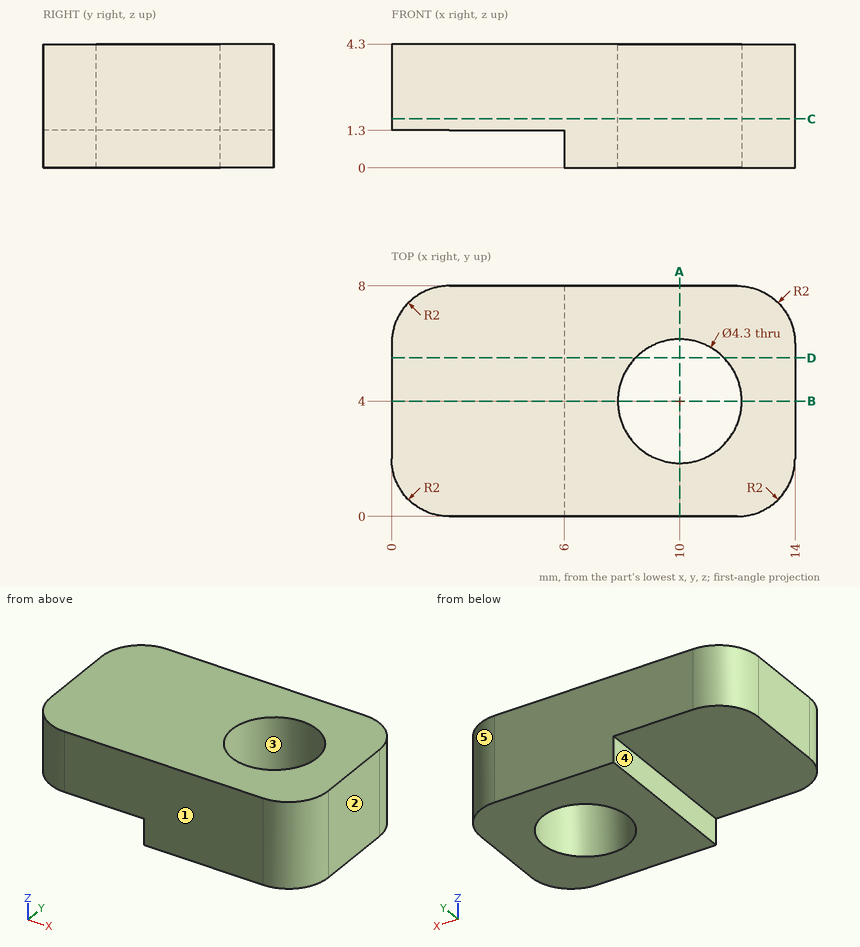
Design review of the part shown in the three views and the two pictorial views. Dimensions are in mm from the part's minimum x, y and z. A direction names the side the tool comes from. Give positions to 0.01 mm unless a question says otherwise; leave off trailing zeros. Loops run counter-clockwise (first coordinate to the right, second up) from the corner with the lowest first, then second, coordinate; pieces in that order, holes last. Notation, with made-up numbers: (67.25, -10) -> (75.25, -10) arc R14 ccw to (75.25, -1) -> close; hole circle Ø5 at (29, 77). An arc over 180 degrees is marked (long way). Write each question's results on one line, items separated by ' | '.
1) Take a section at D-D, the plane y = 5.5. Give the boundary of the cut face in (x, z).
Conclusion:
outline: (0, 1.3) -> (6, 1.3) -> (6, 0) -> (8.46, 0) -> (8.46, 4.3) -> (0, 4.3) -> close; (11.54, 0) -> (14, 0) -> (14, 4.3) -> (11.54, 4.3) -> close
2) For line 1 along Y through (x, z) = (10, 3.1); line 2 along Z through (x, y) = (1.25, 2.5); line 3 along X through (y, z) = (3.25, 1.55), list the stretches that pass through material, from the lowest coordinate up. Write a range as from..to.
Conclusion:
line 1: y = 0..1.85, 6.15..8 | line 2: z = 1.3..4.3 | line 3: x = 0..7.99, 12.01..14
3) Take a section at A-A, the plane x = 10. Give the boundary of the cut face in (y, z).
Conclusion:
outline: (0, 0) -> (1.85, 0) -> (1.85, 4.3) -> (0, 4.3) -> close; (6.15, 0) -> (8, 0) -> (8, 4.3) -> (6.15, 4.3) -> close
4) Take a section at C-C, the plane z = 1.7. Give the boundary of the cut face in (x, y), plus the area to 3 significant figures.
Conclusion:
outline: (0, 2) arc R2 ccw to (2, 0) -> (12, 0) arc R2 ccw to (14, 2) -> (14, 6) arc R2 ccw to (12, 8) -> (2, 8) arc R2 ccw to (0, 6) -> close; hole circle Ø4.3 at (10, 4) | area: 94.0 mm^2
5) Draft analysis for pull direction X (two halves, no side actions). For the marked faces 1, 2 and 3, state which applies: pulls with the +X half, pulls with the -X half, needs draft (parallel to the pull), parting line crosses it, or undercut.
Conclusion:
face 1: needs draft | face 2: pulls with the +X half | face 3: undercut
6) Take a section at B-B, the plane y = 4. Give the boundary of the cut face in (x, z), plus the area to 3 significant figures.
Conclusion:
outline: (0, 1.3) -> (6, 1.3) -> (6, 0) -> (7.85, 0) -> (7.85, 4.3) -> (0, 4.3) -> close; (12.15, 0) -> (14, 0) -> (14, 4.3) -> (12.15, 4.3) -> close | area: 33.9 mm^2
7) Insertion check: pin 1 Ø1.8 at (x, y) = (2, 5) entering from -Z. The pin has a flat end and moves straight along its axis. Give the tip position at first contact, or say it passes through.
Conclusion:
pin 1: stops at z = 1.3
8) Tool access review of the marked faces 4 and 5: name each direction out of +Z, -Z, +X, -X, +Y, -Y from which nothing blocks a thin tool from reaching the whole face with its end or side.
Conclusion:
face 4: -Z, -X, +Y, -Y | face 5: +Z, -Z, +X, +Y
